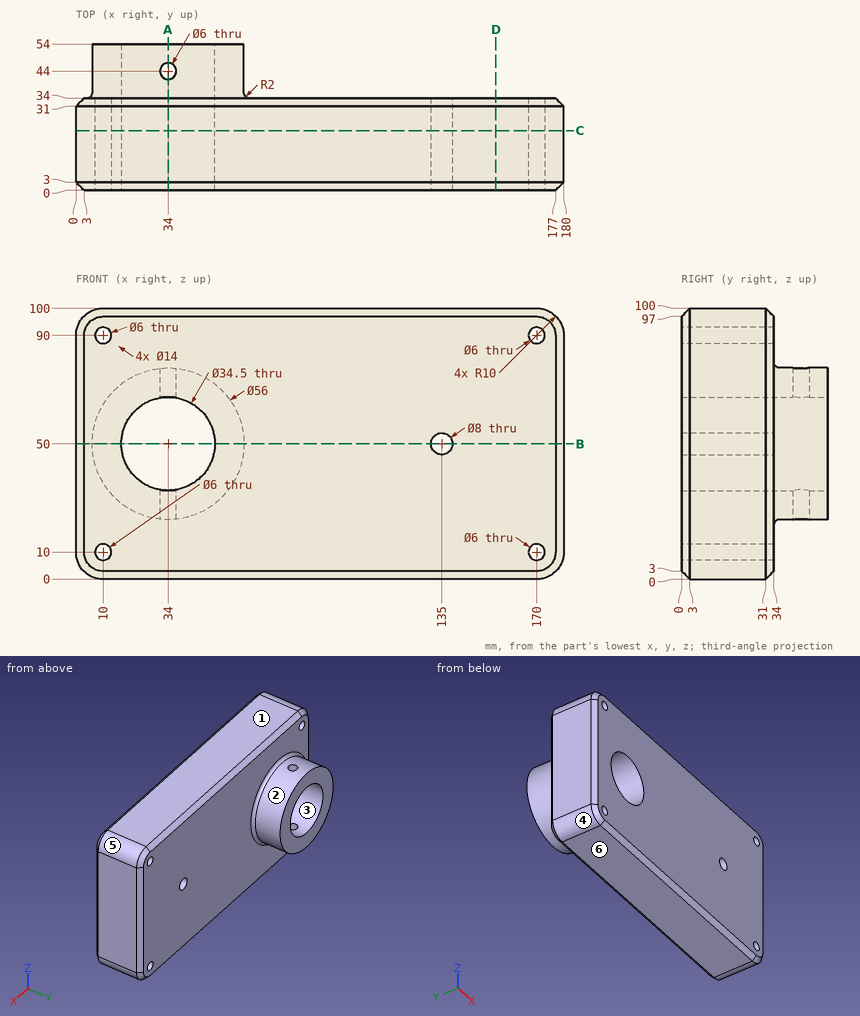
Design review of the part shown in the three views and the two pictorial views. Dimensions are in mm from the part's minimum x, y and z. A direction names the side the tool comes from. Give positions to 0.01 mm unless a question says otherwise; leave off trailing zeros. Loops run counter-clockwise (first coordinate to the right, second up) from the corner with the lowest first, then second, coordinate; pieces in that order, holes last. Notation, with made-up numbers: M -5.75,9.25 L 29.25,9.25 A15 cw 29.25,35.25 Z; hole C 43,-11.75 d9. An arc over 180 degrees is marked long. Put each result on its own line as item: value. Start each with the question number.
(1) For pin 1 (3 mm diameter, centred on y = 16.5, z = 42, fed in from -X); pin 2 (9.5 mm diameter, centred on x = 170, z = 90, fed in from +Y); pin 3 (2 mm diameter, centred on y = 43.5, z = 61, fed in from -X); pin 4 (5 mm diameter, centred on x = 10, z = 10, fed in from -Y), all flat-tipped, find the tip position at first contact; note any pin that passes through.
(2) Add section C-C, the plane y = 22. Write out the cut boundary in (x, z), then the cut area to 3 significant figures.
(3) Machinability: for the marked faces 1 and 2, which of the approach directions +Z, -Z, +X, -X, +Y, -Y give a long, thin tool a straight path to every point of the face, cutting with its end or side? Answer none if there is none.
(4) Add section D-D, the plane x = 155. Write out the cut boundary in (y, z).
(5) Wall thickness on L1, parallel to X at y = 25, z = 10; L2, parallel to Z at x = 170, y = 13; L3, parallel to Y at x = 34, z = 72.75: over which ranges is each line inside the solid? List them lowest first.
(6) Add section B-B, the plane z = 50. Write out the cut boundary in (x, y), then the cut area to 3 significant figures.
(7) Add section A-A, the plane x = 34. Write out the cut boundary in (y, z).
(8) The part is to be moulded in two halves that separate along X. For the marked faces 3, 4, 5 and 6, say which applies: +X half, -X half, draft (parallel to the pull), parting line (faces both ways), or undercut.
Result:
1. pin 1: stops at x = 0
1. pin 2: stops at y = 34
1. pin 3: stops at x = 7.85
1. pin 4: passes through
2. outline: M 0,10 A10 ccw 10,0 L 170,0 A10 ccw 180,10 L 180,90 A10 ccw 170,100 L 10,100 A10 ccw 0,90 Z; hole C 10,10 d6; hole C 10,90 d6; hole C 34,50 d34.5; hole C 135,50 d8; hole C 170,10 d6; hole C 170,90 d6
2. area: 16,800 mm^2
3. face 1: +Z, +X, -X, +Y, -Y
3. face 2: +Y
4. outline: M 0,3 L 3,0 L 31,0 L 34,3 L 34,97 L 31,100 L 3,100 L 0,97 Z
5. L1: x = 0 to 7, 13 to 167, 173 to 180
5. L2: z = 0 to 7, 13 to 87, 93 to 100
5. L3: y = 0 to 41, 47 to 54
6. outline: M 0,3 L 3,0 L 16.75,0 L 16.75,54 L 6,54 L 6,36 A2 cw 4,34 L 3,34 L 0,31 Z; M 51.25,0 L 131,0 L 131,34 L 64,34 A2 cw 62,36 L 62,54 L 51.25,54 Z; M 139,0 L 177,0 L 180,3 L 180,31 L 177,34 L 139,34 Z
6. area: 5,090 mm^2
7. outline: M 0,3 L 3,0 L 31,0 L 34,3 L 34,20 A2 cw 36,22 L 41,22 L 41,32.75 L 0,32.75 Z; M 0,67.25 L 41,67.25 L 41,78 L 36,78 A2 cw 34,80 L 34,97 L 31,100 L 3,100 L 0,97 Z; M 47,22 L 54,22 L 54,32.75 L 47,32.75 Z; M 47,67.25 L 54,67.25 L 54,78 L 47,78 Z
8. face 3: undercut
8. face 4: -X half
8. face 5: +X half
8. face 6: draft
